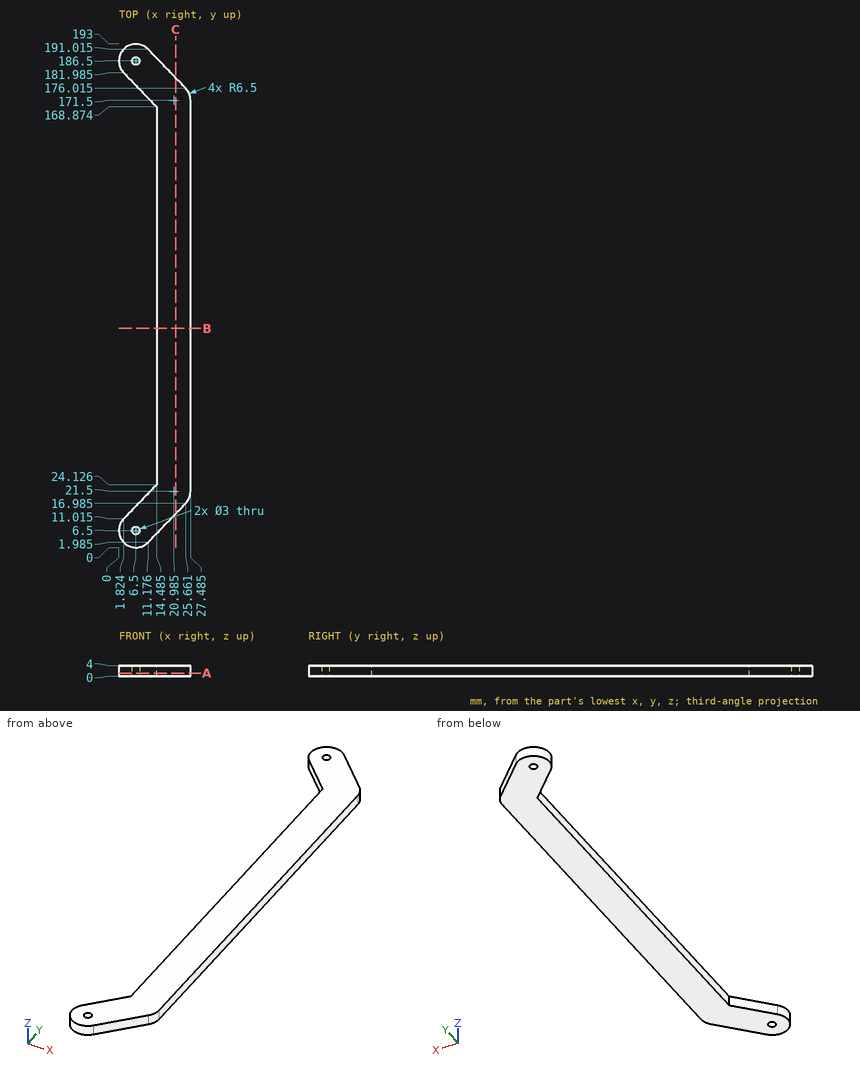
Study the drawing (mm; zero at the part's minimum x, y, z) and answer. Give positions to 0.01 mm unless a question says otherwise; leave off trailing zeros. Write each loop counter-clockwise with the first axis right and the second up, starting at its lowest first coordinate (ties: lowest second). Pieces come first, ordered by that corner, then holes. Notation, with made-up numbers: (62, -29) - (88, -29) arc R31 ccw to (88, 6) - close; hole circle Ø1 at (-17.75, -26). An arc over 180 degrees is marked (long way). One line per question, with ' | ' between items. Start each with the question number.
1. Section B-B, the plane y = 84 is taken. Determine the outline of the cut face in (x, z) (1 decimal).
2. Section A-A, the plane z = 1.1 is taken. Determine the outline of the cut face in (x, y) (1 decimal), then the cut area to 3 significant figures.
3. Section C-C, the plane x = 21.75 is taken. Determine the outline of the cut face in (y, z) (1 decimal).
4. Given P1, Ø2.5, axis at x = 6.5, y = 6.5, coming from the +Z side; P2, Ø1, axis at y = 165, z = 0.5, coming from the -X side (1 decimal); P3, Ø2, axis at x = 15.5, z = 1.5, coming from the -Y side, each flat-ended and moving along its own axis, determine where each tip first touches the part or whether it passes through.
5. Straight lines are drawn through the part: line 1 (Y direction, x = 5.5, z = 2.9); line 2 (Y direction, x = 6.5, z = 1.05); line 3 (X direction, y = 136.5, z = 1.3) (1 decimal). For each, find the intervals that lie inside material, in ascending order.
Result:
1) outline: (14.5, 0) - (27.5, 0) - (27.5, 4) - (14.5, 4) - close
2) outline: (1.8, 11) arc R6.5 ccw to (11.2, 2) - (25.7, 17) arc R6.5 ccw to (27.5, 21.5) - (27.5, 171.5) arc R6.5 ccw to (25.7, 176) - (11.2, 191) arc R6.5 ccw to (1.8, 182) - (14.5, 168.9) - (14.5, 24.1) - close; hole circle Ø3 at (6.5, 6.5); hole circle Ø3 at (6.5, 186.5) | area: 2,610 mm2
3) outline: (12.9, 0) - (180.1, 0) - (180.1, 4) - (12.9, 4) - close
4) P1: passes through | P2: stops at x = 14.5 | P3: stops at y = 5.43
5) line 1: y = 0.08 to 5.38, 7.62 to 14.82, 178.18 to 185.38, 187.62 to 192.92 | line 2: y = 0 to 5, 8 to 15.86, 177.14 to 185, 188 to 193 | line 3: x = 14.5 to 27.5
